Design review of the part built by this model. Coordinates are the model's own, in mm. A direction names the side the tool comes from. Coordinates: 2 decimals unless noted, no trailing zeros. Loops run counter-clockwise (first coordinate to the right, second up) from the corner with the lowest first, then second, coordinate; pieces in that order, holes last. Notation, with made-up numbers: (62.5, 16) -> (83.5, 16) arc R27 cw to (83.5, 51) -> close; hole circle Ø11 at (72.25, 67.5). An arc over 180 degrees is marked (long way). Answer as a JSON object with one key per item and string values.
```python
from build123d import *

# Parameters (mm, degrees)
F0_W          = 10
F0_H          = 7
F0_W_2        = 7
F0_H_2        = 28
F1_DEPTH      = 20
F2_R          = 3.5
F2_R_2        = 1.75
F3_DEPTH      = 3.3
F4_DEPTH      = 25
F6_DEPTH      = 3.3
F7_DEPTH      = 25
F9_DEPTH      = 25
F10_SIZE      = 7
F11_T1_DEPTH  = 35.4300979278
F12_SIZE      = 6.99999
F13_T1_DEPTH  = 7
F13_T6_DEPTH  = 29.9594705668
F13_T11_DEPTH = 29.9594705668
F13_T16_DEPTH = 29.9594705668
F13_T21_DEPTH = 29.9594705668
F14_T1_DEPTH  = 26.1433659759
F14_T3_DEPTH  = 20.1862268885
F14_T5_DEPTH  = 20.1862268885
F14_T10_DEPTH = 38.2867219519
F14_T15_DEPTH = 38.2867219519
F14_T20_DEPTH = 38.2867219519
F14_T25_DEPTH = 38.2867219519
F15_SIZE      = 2
F16_SIZE      = 2


# Not quite as in the source:
# - a fillet or chamfer that OpenCascade refuses, or shapes differently, is made with other operations: its cross-section is extruded or revolved along the edge and cut away or added
# - a fillet or chamfer is up to 0.001 mm smaller than in the source, because OpenCascade refuses the exact size


with BuildPart() as f1:
    # F0 (on Front) → F1 (new body)
    with BuildSketch(Plane.XZ):
        with Locations((-15.5, 3.5)):
            Rectangle(F0_W, F0_H)
        with Locations((-7, 3.5)):
            Rectangle(F0_W_2, F0_H)
        with Locations((0, 3.5)):
            Rectangle(F0_W_2, F0_H)
        with Locations((-7, 21)):
            Rectangle(F0_W_2, F0_H_2)
        with Locations((7, 3.5)):
            Rectangle(F0_W_2, F0_H)
        with Locations((15.5, 3.5)):
            Rectangle(F0_W, F0_H)
        with Locations((7, 21)):
            Rectangle(F0_W_2, F0_H_2)
    extrude(amount=F1_DEPTH)

    # F2 (on face) → F3 (cut)
    with BuildSketch(Plane.XY.offset(7)):
        with Locations((15.5, -10)):
            Circle(F2_R)
        with Locations((15.5, -10)):
            Circle(F2_R_2, mode=Mode.SUBTRACT)
    extrude(amount=-F3_DEPTH, mode=Mode.SUBTRACT)

    # F2 (on face) → F4 (cut)
    with BuildSketch(Plane.XY.offset(7)):
        with Locations((15.5, -10)):
            Circle(F2_R_2)
    extrude(amount=-F4_DEPTH, mode=Mode.SUBTRACT)

    # F5 (on face) → F6 (cut)
    with BuildSketch(Plane.XY.offset(7)):
        with BuildLine():
            ThreePointArc((-12, -10), (-15.5, -6.5), (-19, -10))
            ThreePointArc((-19, -10), (-15.5, -13.5), (-12, -10))
        make_face()
        with BuildLine():
            ThreePointArc((-13.75, -10), (-15.5, -11.75), (-17.25, -10))
            ThreePointArc((-17.25, -10), (-15.5, -8.25), (-13.75, -10))
        make_face(mode=Mode.SUBTRACT)
    extrude(amount=-F6_DEPTH, mode=Mode.SUBTRACT)

    # F7 (cut): a face of the model
    f7_faces = [f1.faces().sort_by_distance(p)[0] for p in [
        (-15.5, -10, 7),
    ]]
    extrude(f7_faces, amount=-F7_DEPTH, mode=Mode.SUBTRACT)

    # F8 (on face) → F9 (cut)
    with BuildSketch(Plane(origin=(-10.5, 0, 0), x_dir=(0, -1, 0), z_dir=(-1, 0, 0))):
        with BuildLine():
            ThreePointArc((10, 31.75), (8.7625631329, 28.7625631329), (11.75, 30))
            ThreePointArc((11.75, 30), (11.2374368671, 31.2374368671), (10, 31.75))
        make_face()
    extrude(amount=-F9_DEPTH, mode=Mode.SUBTRACT)

    # F10
    f10_edges = [f1.edges().sort_by_distance(p)[0] for p in [
        (-7, -20, 35),
        (-7, 0, 35),
        (7, 0, 35),
        (7, -20, 35),
    ]]
    chamfer(f10_edges, length=F10_SIZE)

    # F11: chamfer of 3 on 2 edges, made by hand

    # F11_s2 → F11_t1 (cut)
    with BuildSketch(Plane.XZ.offset(-7.7150489639)):
        Polygon((17.5, 7), (20.5, 4), (20.5, 7), align=None)
        Polygon((-20.5, 4), (-17.5, 7), (-20.5, 7), align=None)
    extrude(amount=F11_T1_DEPTH, mode=Mode.SUBTRACT)

    # F12 (size 7 in the source; OpenCascade refuses exactly that, so slightly less here)
    f12_edges = [f1.edges().sort_by_distance(p)[0] for p in [
        (0, 0, 7),
        (0, -20, 7),
    ]]
    chamfer(f12_edges, length=F12_SIZE)

    # F13: chamfer of 5 on 6 edges, made by hand

    # F13_s2 → F13_t1 (cut)
    with BuildSketch(Plane.YZ.offset(-3.5)):
        Polygon((-5.5355239059, 5.5355339059), (-9.0710578119, 7), (-6.99999, 7), align=None)
        Polygon((-10.9289421881, 7), (-14.4644760941, 5.5355339059), (-13.00001, 7), align=None)
    extrude(amount=F13_T1_DEPTH, mode=Mode.SUBTRACT)


with BuildPart() as f13_tool4:
    # F13_s5 → F13_t6 (new body)
    with BuildSketch(Plane(origin=(17.3422723993, 0, -17.3422723993), x_dir=(0, 1, 0), z_dir=(-0.7071067812, 0, 0.7071067812))):
        Polygon((-15, -17.3241161391), (-20, -12.3241161391), (-20, -17.3241161391), align=None)
    extrude(amount=F13_T6_DEPTH)

    split(bisect_by=Plane.XY.offset(7), keep=Keep.BOTTOM)


with BuildPart() as f1_1:
    add(f1.part)

    # F13_t3: cut F13_tool4
    add(f13_tool4.part, mode=Mode.SUBTRACT)


with BuildPart() as f13_tool9:
    # F13_s10 → F13_t11 (new body)
    with BuildSketch(Plane(origin=(17.3422723993, 0, -17.3422723993), x_dir=(0, 1, 0), z_dir=(-0.7071067812, 0, 0.7071067812))):
        Polygon((0, -12.3241161391), (-5, -17.3241161391), (0, -17.3241161391), align=None)
    extrude(amount=F13_T11_DEPTH)

    split(bisect_by=Plane.XY.offset(7), keep=Keep.BOTTOM)


with BuildPart() as f1_2:
    add(f1_1.part)

    # F13_t8: cut F13_tool9
    add(f13_tool9.part, mode=Mode.SUBTRACT)


with BuildPart() as f13_tool14:
    # F13_s15 → F13_t16 (new body)
    with BuildSketch(Plane(origin=(3.8422723993, 0, 3.8422723993), x_dir=(0, 1, 0), z_dir=(-0.7071067812, 0, -0.7071067812))):
        Polygon((0, -12.3241161391), (-5, -17.3241161391), (0, -17.3241161391), align=None)
    extrude(amount=F13_T16_DEPTH)

    split(bisect_by=Plane.XY.offset(7), keep=Keep.BOTTOM)


with BuildPart() as f1_3:
    add(f1_2.part)

    # F13_t13: cut F13_tool14
    add(f13_tool14.part, mode=Mode.SUBTRACT)


with BuildPart() as f13_tool19:
    # F13_s20 → F13_t21 (new body)
    with BuildSketch(Plane(origin=(3.8422723993, 0, 3.8422723993), x_dir=(0, 1, 0), z_dir=(-0.7071067812, 0, -0.7071067812))):
        Polygon((-15, -17.3241161391), (-20, -12.3241161391), (-20, -17.3241161391), align=None)
    extrude(amount=F13_T21_DEPTH)

    split(bisect_by=Plane.XY.offset(7), keep=Keep.BOTTOM)


with BuildPart() as f1_4:
    add(f1_3.part)

    # F13_t18: cut F13_tool19
    add(f13_tool19.part, mode=Mode.SUBTRACT)

    # F14: chamfer of 2 on 16 edges, made by hand

    # F14_s2 → F14_t1 (cut)
    with BuildSketch(Plane.XY.offset(7)):
        Polygon((-10.5, -18), (-8.5, -20), (-10.5, -20), align=None)
        Polygon((10.5, -18), (8.5, -20), (10.5, -20), align=None)
        Polygon((8.5, 0), (10.5, -2), (10.5, 0), align=None)
        Polygon((-8.5, 0), (-10.5, -2), (-10.5, 0), align=None)
    extrude(amount=F14_T1_DEPTH, mode=Mode.SUBTRACT)

    # F14_s4 → F14_t3 (cut)
    with BuildSketch(Plane(origin=(0, 0.3630910403, 0.3630910403), x_dir=(1, 0, 0), z_dir=(0, 0.7071067812, 0.7071067812))):
        Polygon((10.5, -31.941125497), (8.5, -33.941125497), (10.5, -33.941125497), align=None)
        Polygon((3.5, -31.941125497), (5.5, -33.941125497), (3.5, -33.941125497), align=None)
        Polygon((-10.5, -31.941125497), (-8.5, -33.941125497), (-10.5, -33.941125497), align=None)
        Polygon((-3.5, -31.941125497), (-5.5, -33.941125497), (-3.5, -33.941125497), align=None)
    extrude(amount=F14_T3_DEPTH, mode=Mode.SUBTRACT)

    # F14_s6 → F14_t5 (cut)
    with BuildSketch(Plane(origin=(0, -10.3630910403, 10.3630910403), x_dir=(1, 0, 0), z_dir=(0, -0.7071067812, 0.7071067812))):
        Polygon((3.5, 17.7989898732), (5.5, 19.7989898732), (3.5, 19.7989898732), align=None)
        Polygon((8.5, 19.7989898732), (10.5, 17.7989898732), (10.5, 19.7989898732), align=None)
        Polygon((-5.5, 19.7989898732), (-3.5, 17.7989898732), (-3.5, 19.7989898732), align=None)
        Polygon((-10.5, 17.7989898732), (-8.5, 19.7989898732), (-10.5, 19.7989898732), align=None)
    extrude(amount=F14_T5_DEPTH, mode=Mode.SUBTRACT)


with BuildPart() as f14_tool8:
    # F14_s9 → F14_t10 (new body)
    with BuildSketch(Plane.XY.offset(33.1433659759)):
        Polygon((-3.5, -18), (-5.5, -20), (-3.5, -20), align=None)
    extrude(amount=-F14_T10_DEPTH)

    split(bisect_by=Plane(origin=(0, -10.000005, 10.000005), x_dir=(1, 0, 0), z_dir=(0, -0.7071067812, 0.7071067812)), keep=Keep.TOP)


with BuildPart() as f1_5:
    add(f1_4.part)

    # F14_t7: cut F14_tool8
    add(f14_tool8.part, mode=Mode.SUBTRACT)


with BuildPart() as f14_tool13:
    # F14_s14 → F14_t15 (new body)
    with BuildSketch(Plane.XY.offset(-5.1433559759)):
        Polygon((3.5, -18), (5.5, -20), (3.5, -20), align=None)
    extrude(amount=F14_T15_DEPTH)

    split(bisect_by=Plane(origin=(0, -10.000005, 10.000005), x_dir=(1, 0, 0), z_dir=(0, -0.7071067812, 0.7071067812)), keep=Keep.TOP)


with BuildPart() as f1_6:
    add(f1_5.part)

    # F14_t12: cut F14_tool13
    add(f14_tool13.part, mode=Mode.SUBTRACT)


with BuildPart() as f14_tool18:
    # F14_s19 → F14_t20 (new body)
    with BuildSketch(Plane.XY.offset(-5.1433559759)):
        Polygon((5.5, 0), (3.5, -2), (3.5, 0), align=None)
    extrude(amount=F14_T20_DEPTH)

    split(bisect_by=Plane(origin=(0, 5e-06, 5e-06), x_dir=(1, 0, 0), z_dir=(0, 0.7071067812, 0.7071067812)), keep=Keep.TOP)


with BuildPart() as f1_7:
    add(f1_6.part)

    # F14_t17: cut F14_tool18
    add(f14_tool18.part, mode=Mode.SUBTRACT)


with BuildPart() as f14_tool23:
    # F14_s24 → F14_t25 (new body)
    with BuildSketch(Plane.XY.offset(33.1433659759)):
        Polygon((-5.5, 0), (-3.5, -2), (-3.5, 0), align=None)
    extrude(amount=-F14_T25_DEPTH)

    split(bisect_by=Plane(origin=(0, 5e-06, 5e-06), x_dir=(1, 0, 0), z_dir=(0, 0.7071067812, 0.7071067812)), keep=Keep.TOP)


with BuildPart() as f1_8:
    add(f1_7.part)

    # F14_t22: cut F14_tool23
    add(f14_tool23.part, mode=Mode.SUBTRACT)

    # F15
    f15_edges = [f1_8.edges().sort_by_distance(p)[0] for p in [
        (10.5, -10, 35),
        (3.5, -10, 35),
        (-3.5, -10, 35),
        (-10.5, -10, 35),
    ]]
    chamfer(f15_edges, length=F15_SIZE)

    # F16
    f16_edges = [f1_8.edges().sort_by_distance(p)[0] for p in [
        (-9.464466, 0, 7),
        (9.464466, 0, 7),
        (-9.464466, -20, 7),
        (9.464466, -20, 7),
    ]]
    chamfer(f16_edges, length=F16_SIZE)


solid = f1_8.part
```
1) For faces 5 (the flat face through (-15, -8, 3.7)), 6 (the flat face through (-11.6, -9.9, 7)), 7 (the flat face through (4.5, -10, 34)), 8 (the flat face through (-9.5, -19, 16.3)), 9 (the flat face through (-4.5, -1, 14.2)), list the 3-axis set-ups (+Z, -Z, +X, -X, +Y, -Y) from which the entire face can be reached by the end or side of a thin tool; tool diameter is ignored.
Completed:
{"face 5": "+Z", "face 6": "+Z, -X, +Y, -Y", "face 7": "+Z, +Y, -Y", "face 8": "+Z, -X, -Y", "face 9": "+Z, +Y"}
2) Wall thickness on probe 1 along X at (y, z) = (-18, 13); probe 2 along Y at (x, z) = (-5.5, 30); probe 3 along Z at (x, y) = (-13.5, -11.5): over which ranges is each line inside the solid? List them lowest first.
Completed:
{"probe 1": "-10.5 to -3.5, 3.5 to 10.5", "probe 2": "-18 to -11.75, -8.25 to -2", "probe 3": "0 to 3.7"}
3) Clearance check with flat-ended pins moving along their axes: pin 1 Ø4.5 at (y, z) = (-10, 30) entering from +X; pin 2 Ø1.5 at (x, y) = (-1, -10) entering from +Z; pin 3 Ø4 at (x, z) = (5.5, 30.5) entering from +Y. State where each tip first meets the part, or that it passes through.
Completed:
{"pin 1": "x = 10.5", "pin 2": "z = 7", "pin 3": "y = -0.5"}
4) The part is to be moulded in two halves that separate along Y. For faces 1 (the flat face through (17.2, -2.47, 3.72)), 2 (the flat face through (17.25, -17.46, 3.77)), 3 (the cylindrical face through (-12, -10, 5)), 4 (the cylindrical face through (12, -10, 5)), say which applies: pulls with the +Y half, pulls with the -Y half, needs draft (parallel to the pull), parting line crosses it, or undercut.
Completed:
{"face 1": "pulls with the +Y half", "face 2": "pulls with the -Y half", "face 3": "undercut", "face 4": "undercut"}
5) Add section A-A, the plane z = 9.5. Give the boundary of the cut face in (x, y), and give its area (3 significant figures).
Completed:
{"outline": "(-10.5, -18) -> (-8.5, -20) -> (-5.5, -20) -> (-3.5, -18) -> (-3.5, -2) -> (-5.5, 0) -> (-8.5, 0) -> (-10.5, -2) -> close; (3.5, -18) -> (5.5, -20) -> (8.5, -20) -> (10.5, -18) -> (10.5, -2) -> (8.5, 0) -> (5.5, 0) -> (3.5, -2) -> close", "area": "264 mm²"}
6) Add section C-C, the plane x = 8. Give the boundary of the cut face in (y, z), and give its area (3 significant figures).
Completed:
{"outline": "(-20, 0) -> (0, 0) -> (0, 28) -> (-7, 35) -> (-13, 35) -> (-20, 28) -> close; hole circle Ø3.5 at (-10, 30)", "area": "641 mm²"}
7) Add section D-D, the plane z = 4.5. Give the boundary of the cut face in (x, y).
Completed:
{"outline": "(-20, -15) -> (-12.93, -20) -> (-5.5, -20) -> (-3.5, -18) -> (-3.5, -15.5) -> (3.5, -15.5) -> (3.5, -18) -> (5.5, -20) -> (12.93, -20) -> (20, -15) -> (20, -5) -> (12.93, 0) -> (5.5, 0) -> (3.5, -2) -> (3.5, -4.5) -> (-3.5, -4.5) -> (-3.5, -2) -> (-5.5, 0) -> (-12.93, 0) -> (-20, -5) -> close; hole circle Ø7 at (-15.5, -10); hole circle Ø7 at (15.5, -10)"}
